Part print with two shaded views. Sizes in mm from the minimum x, y, z corner. A direction names the side the tool comes from. Round coordinates to 2 decimals unless told otherwise and drop trailing zeros. Loops run counter-clockwise (first coordinate to the right, second up) from the corner with the lowest first, then second, coordinate; pieces in that order, holes last. Notation, with made-up numbers: M 39.25,4 L 88.25,4 A14 ccw 88.25,8 Z; hole C -34.5,-40 d4. An arc over 180 degrees is marked long. Use a Markdown table: item, result. Add a question column.
Item 1: Wall check: L1, parallel to Y at x = 13, z = 4.25 (1 decimal); L2, parallel to X at y = 1.9, z = 0.5 (1 decimal); L3, parallel to X at y = 1.5, z = 4.5 (1 decimal). Give the ranges that are in metal, low to high. Write a range as from..to.
Item 2: Saw through at C-C on x = 8.25. Write the cut outline in (y, z).
Item 3: Saw through at B-B on z = 3.25. Write the cut outline in (x, y) (1 decimal).
Item 4: Saw through at D-D on z = 6. Write the cut outline in (x, y) (1 decimal).
Item 5: Saw through at A-A on y = 0.8. Write the cut outline in (x, z) (1 decimal).
Item 6: Two-plate mould, pull along Y, no slides. Class the marked faces 1, 2, 3 and 4: +Y half, -Y half, draft (parallel to the pull), parting line (faces both ways), or undercut.
Item 7: Tool access for the marked faces 5 and 6: list every direction of +Z, -Z, +X, -X, +Y, -Y with a clear straight run to the whole face (end or side of a thin tool).
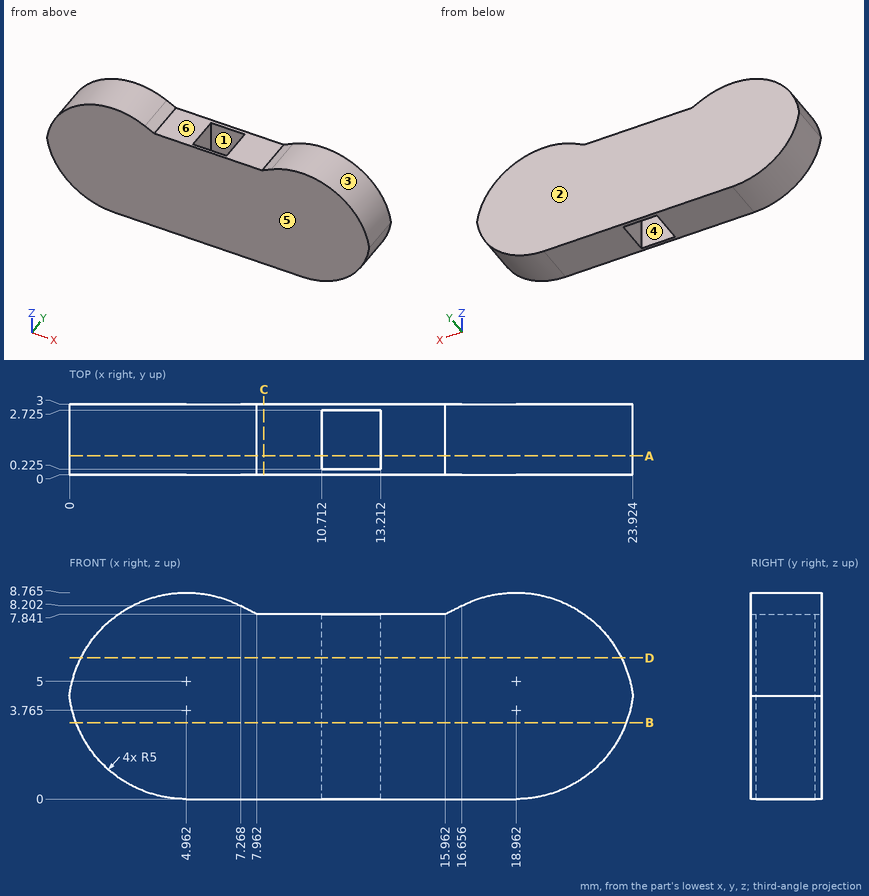
Entries:
| question | item | result |
|---|---|---|
| 1 | L1 | 0..0.2, 2.7..3 |
| 1 | L2 | 2.8..10.7, 13.2..21.1 |
| 1 | L3 | 0..10.7, 13.2..23.9 |
| 2 | outline | M 0,0 L 3,0 L 3,7.84 L 0,7.84 Z |
| 3 | outline | M 0.3,0 L 23.6,0 L 23.6,3 L 0.3,3 Z; hole M 10.7,0.2 L 13.2,0.2 L 13.2,2.7 L 10.7,2.7 Z |
| 4 | outline | M 0.5,0 L 23.4,0 L 23.4,3 L 0.5,3 Z; hole M 10.7,0.2 L 13.2,0.2 L 13.2,2.7 L 10.7,2.7 Z |
| 5 | outline | M 0,4.4 A5 ccw 5,0 L 10.7,0 L 10.7,7.8 L 8,7.8 L 7.3,8.2 A5 ccw Z; M 13.2,0 L 19,0 A5 ccw 23.9,4.4 A5 ccw 16.7,8.2 L 16,7.8 L 13.2,7.8 Z |
| 6 | face 1 | undercut |
| 6 | face 2 | +Y half |
| 6 | face 3 | draft |
| 6 | face 4 | undercut |
| 7 | face 5 | +Z, -Z, +X, -X, -Y |
| 7 | face 6 | +Z, +Y, -Y |
